Check sheet for the modelled part. Datum: model origin and axes. Units: mm. Give positions to 0.01 mm unless a question says otherwise; leave off trailing zeros. Order: outer loops, then holes, each group sorted by start corner. A loop starts at its lowest first (then second) coordinate and runs counter-clockwise, first axis right, second up.
Item 1: Material ranges on line 1 along Y through (x, z) = (69.5, -0.8); line 2 along X through (y, z) = (20.5, 2.15); line 3 along Y through (x, z) = (24.5, 0.5), recorded low to high.
Item 2: Sectioned sample at C-C on x = 71.5. Record the boundary of the cut face in (y, z), and give its area (3 significant figures).
Item 3: Gauge pin test, flat end, axial feed: P1, Ø2.5, axis at x = 70.5, z = 0.5, coming from the +Y side. Record the tip position at first contact, or that the pin passes through.
Item 4: Sectioned sample at B-B on z = 0.15. Record the boundary of the cut face in (x, y), and give its area (3 significant figures).
Item 5: Sectioned sample at A-A on y = 9.5. Record the boundary of the cut face in (x, z), and give its area (3 significant figures).
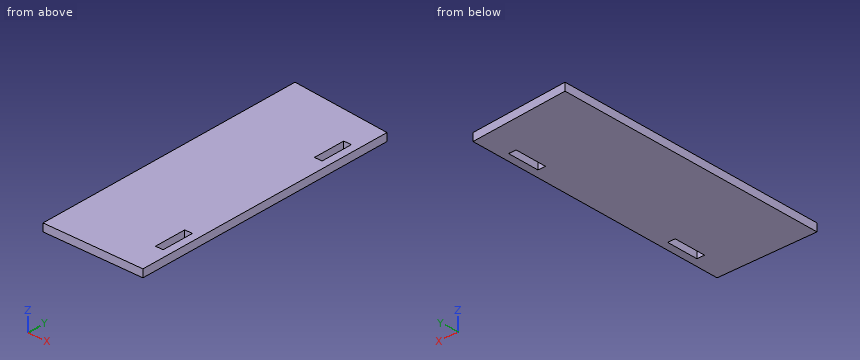
Autodesk Inventor part; units mm, degrees
ref_plane "YZ Plane" through (0, 0, 0) normal (1, 0, 0) x (0, 1, 0)
ref_plane "XZ Plane" through (0, 0, 0) normal (0, 1, 0) x (-1, 0, 0)
ref_plane "XY Plane" through (0, 0, 0) normal (0, 0, 1) x (1, 0, 0)
sketch "Sketch1" plane through (0, 0, 0) normal (0, 0, 1) x (1, 0, 0)
  line L0 (14.1765, -18.066) -> (14.1765, 162.6208)
  line L1 (14.1765, -18.066) -> (79.1765, -18.066)
  line L2 (79.1765, -18.066) -> (79.1765, 156.934)
  line L3 (79.1765, -18.066) -> (14.1765, -18.066)
  line L4 (79.1765, -18.066) -> (14.1765, -18.066)
  line L5 (14.1765, 162.6208) -> (79.1765, 156.934)
  line L6 (79.1765, 136.934) -> (74.1765, 136.934)
  line L7 (74.1765, 136.934) -> (74.1765, 115.934)
  line L8 (74.1765, 115.934) -> (79.1765, 115.934)
  line L9 (79.1765, 115.934) -> (79.1765, 136.934)
  line L10 (69.1765, 22.934) -> (74.1765, 22.934)
  line L11 (74.1765, 22.934) -> (74.1765, 1.934)
  line L12 (74.1765, 1.934) -> (69.1765, 1.934)
  line L13 (69.1765, 1.934) -> (69.1765, 22.934)
  line L14 (74.1765, 136.934) -> (69.1765, 136.934)
  line L15 (69.1765, 136.934) -> (69.1765, 115.934)
  line L16 (69.1765, 115.934) -> (74.1765, 115.934)
  line L17 (74.1765, 115.934) -> (74.1765, 136.934)
  point P0 (0, 0)
  point P1 (71.6765, 1.934)
  point P2 (79.2985, 0.69)
  point P3 (79.2985, 20.69)
  point P4 (79.1765, 115.934)
  dimension "d3" = 65
  dimension "d23" = 85
  dimension "d26" = 175
  dimension "d27" = 180.6868
  dimension "d28" = 5
  dimension "d29" = 21
  dimension "d30" = 5
  dimension "d31" = 21
  dimension "d32" = 20
  dimension "d33" = 20
  dimension "d35" = 5
  dimension "d36" = 5
extrude "Extrusion1" add sketch "Sketch1" along normal mid plane 5 contours L0 L5 L2 L6 L14 L15 L16 L8 L1 | L8 L7 L6 L2
equation "\"BendRadius\" = Thickness"
equation "\"BendReliefWidth\" = Thickness"
equation "\"BendReliefDepth\" = 0.5 * Thickness"
equation "\"CornerReliefSize\" = 4 * Thickness"
equation "\"MinimumRemnant\" = 2 * Thickness"
equation "\"TransitionRadius\" = BendRadius"
equation "\"JacobiRadiusSize\" = BendRadius"
equation "\"GapSize\" = Thickness"
properties part number "standformiddleslide1"
Report:
1. line 1: y = -18.07 to 1.93, 22.93 to 115.93, 136.93 to 157.78
1. line 2: x = 14.18 to 69.18, 74.18 to 79.18
1. line 3: y = -18.07 to 161.72
2. outline: (-18.07, -2.5) - (1.93, -2.5) - (1.93, 2.5) - (-18.07, 2.5) - close; (22.93, -2.5) - (115.93, -2.5) - (115.93, 2.5) - (22.93, 2.5) - close; (136.93, -2.5) - (157.61, -2.5) - (157.61, 2.5) - (136.93, 2.5) - close
2. area: 668 mm2
3. P1: stops at y = 157.8
4. outline: (14.18, -18.07) - (79.18, -18.07) - (79.18, 156.93) - (14.18, 162.62) - close; hole (69.18, 1.93) - (74.18, 1.93) - (74.18, 22.93) - (69.18, 22.93) - close; hole (69.18, 115.93) - (74.18, 115.93) - (74.18, 136.93) - (69.18, 136.93) - close
4. area: 11,300 mm2
5. outline: (14.18, -2.5) - (69.18, -2.5) - (69.18, 2.5) - (14.18, 2.5) - close; (74.18, -2.5) - (79.18, -2.5) - (79.18, 2.5) - (74.18, 2.5) - close
5. area: 300 mm2
